Geometry check sheet. Reference: the model listing, model coordinates, mm. A direction names the side the tool comes from. Round coordinates to 2 decimals unless told otherwise and drop trailing zeros. Order: outer loops, then holes, each group sorted by start corner. A loop starts at its lowest first (then second) coordinate and runs counter-clockwise, first axis right, second up.
(1) Sectioned sample at B-B (x = -21.5). Record the boundary of the cut face in (y, z) (1 decimal).
(2) Material ranges on line 1 along X through (y, z) = (12.25, -2); line 2 along Z through (x, y) = (-12.5, 1.75); line 3 along Y through (x, z) = (-1, -0.5) (1 decimal), recorded low to high.
(3) Sectioned sample at A-A (x = 11). Record the boundary of the cut face in (y, z) (1 decimal).
(4) Release check for a two-part mould opening along Z. For faces 1 (the face through (-22.86, 2, -5)), 2 (the face through (0, 25.4, -9)), 3 (the face through (0, 13, 12.7)), 4 (the face through (-22.06, 24.62, -9.27)) record: +Z half, -Z half, draft (parallel to the pull), parting line (faces both ways), or undercut.
(5) Set-up check for faces 5 (the face through (-21.867, 1.61, -9.218)), 6 (the face through (-20.326, 24.617, 8.73)), 7 (the face through (-0.2, 13.95, -4.56)): record each of +Z, -Z, +X, -X, +Y, -Y from which the full face is reachable in a straight line by a thin tool's end or side.
(6) Go/stop test with flat-tipped pins: pin 1 (10 mm diameter, centred on x = -7.5, z = -2, fed in from -Y) (3 decimals); pin 2 (1.5 mm diameter, centred on x = 6.65, z = -0.77, fed in from +Y); pin 3 (0.9 mm diameter, centred on x = -24.5, y = 2, fed in from +Z). Record where each tip stops, or that it passes through.
from build123d import *

# Parameters (mm, degrees)
SKETCH1_W           = 50.8
SKETCH1_H           = 25.4
BOSS_EXTRUDE1_DEPTH = 25.4
SKETCH6_R           = 0.635
CUT_EXTRUDE1_DEPTH  = 39.1
CUT_EXTRUDE2_DEPTH  = 1.5875
CUT_EXTRUDE3_DEPTH  = 3.175
FILLET1_R           = 3.302
FILLET2_R           = 0.8128
CHAMFER1_SIZE       = 0.635
FILLET3_R           = 1.5875


with BuildPart() as part:
    # Sketch1 → Boss-Extrude1 (new body)
    with BuildSketch(Plane(origin=(0, 0, 0), x_dir=(1, 0, 0), z_dir=(0, 1, 0))):
        Rectangle(SKETCH1_W, SKETCH1_H)
    extrude(amount=BOSS_EXTRUDE1_DEPTH)

    # Sketch6 → Cut-Extrude1 (cut, through all)
    with BuildSketch(Plane(origin=(0, 25.4, 0), x_dir=(1, 0, 0), z_dir=(0, 1, 0))):
        with Locations(Location((-5.6134, 1.4605, 0), (0, 0, 270))):
            Circle(SKETCH6_R)
        with Locations(Location((-0.2286, 3.9243, 0), (0, 0, 270))):
            Circle(SKETCH6_R)
        with Locations(Location((-0.2032, 2.3241, 0), (0, 0, 270))):
            Circle(SKETCH6_R)
        with Locations(Location((-4.1402, -5.0927, 0), (0, 0, 270))):
            Circle(SKETCH6_R)
        with Locations(Location((-8.7376, -5.3467, 0), (0, 0, 270))):
            Circle(SKETCH6_R)
        with Locations(Location((6.6548, 0.7747, 0), (0, 0, 270))):
            Circle(SKETCH6_R)
        with Locations(Location((8.2804, 3.1369, 0), (0, 0, 270))):
            Circle(SKETCH6_R)
        with Locations(Location((-3.3782, 0.0635, 0), (0, 0, 270))):
            Circle(SKETCH6_R)
    extrude(amount=-CUT_EXTRUDE1_DEPTH, mode=Mode.SUBTRACT)

    # Sketch7 → Cut-Extrude2 (cut)
    with BuildSketch(Plane(origin=(0, 25.4, 0), x_dir=(1, 0, 0), z_dir=(0, 1, 0))):
        with BuildLine():
            Line((-20.955, -7.024066704), (-20.955, 7.024066704))
            Line((-20.955, 7.024066704), (-22.046716648, 8.115783352))
            ThreePointArc((-22.046716648, 8.115783352), (-22.046716648, 9.283216648), (-20.879283352, 9.283216648))
            Line((-20.879283352, 9.283216648), (-19.787566704, 8.1915))
            Line((-19.787566704, 8.1915), (20.168566704, 8.1915))
            Line((20.168566704, 8.1915), (21.260283352, 9.283216648))
            ThreePointArc((21.260283352, 9.283216648), (22.427716648, 9.283216648), (22.427716648, 8.115783352))
            Line((22.427716648, 8.115783352), (21.336, 7.024066704))
            Line((21.336, 7.024066704), (21.336, -7.024066704))
            Line((21.336, -7.024066704), (22.427716648, -8.115783352))
            ThreePointArc((22.427716648, -8.115783352), (22.427716648, -9.283216648), (21.260283352, -9.283216648))
            Line((21.260283352, -9.283216648), (20.168566704, -8.1915))
            Line((20.168566704, -8.1915), (-19.787566704, -8.1915))
            Line((-19.787566704, -8.1915), (-20.879283352, -9.283216648))
            ThreePointArc((-20.879283352, -9.283216648), (-22.046716648, -9.283216648), (-22.046716648, -8.115783352))
            Line((-22.046716648, -8.115783352), (-20.955, -7.024066704))
        make_face()
    extrude(amount=-CUT_EXTRUDE2_DEPTH, mode=Mode.SUBTRACT)

    # Sketch8 → Cut-Extrude3 (cut)
    with BuildSketch(Plane.XZ):
        Polygon((22.86, 10.16), (-22.86, 10.16), (-22.86, 3.175), (-25.4, 3.175), (-25.4, -3.175), (-22.86, -3.175), (-22.86, -10.16), (22.86, -10.16), align=None)
    extrude(amount=-CUT_EXTRUDE3_DEPTH, mode=Mode.SUBTRACT)

    # Fillet1
    fillet1_edges = [part.edges().sort_by_distance(p)[0] for p in [
        (22.86, 1.5875, 10.16),
        (22.86, 1.5875, -10.16),
        (-22.86, 1.5875, -10.16),
        (-22.86, 1.5875, 10.16),
    ]]
    fillet(fillet1_edges, radius=FILLET1_R)

    # Fillet2
    fillet2_edges = [part.edges().sort_by_distance(p)[0] for p in [
        (-22.86, 1.5875, -3.175),
        (-22.86, 1.5875, 3.175),
    ]]
    fillet(fillet2_edges, radius=FILLET2_R)

    # Chamfer1
    # the kernel refuses this chamfer: 0.635 mm, written as the material it takes off along each edge
    with BuildSketch(Plane(origin=(-5.6134, 3.175, -1.4605), x_dir=(0, 0, 1), z_dir=(-1, 0, 0))) as chamfer1_piece_1:
        Polygon((0.635 + CHAMFER1_SIZE, 0), (0.635, CHAMFER1_SIZE), (0.635, 0), align=None)
    revolve(axis=Axis((-5.6134, 3.175, -1.4605), (0, 1, 0)), mode=Mode.SUBTRACT)
    with BuildSketch(Plane(origin=(-0.2286, 3.175, -3.9243), x_dir=(0, 0, 1), z_dir=(-1, 0, 0))) as chamfer1_piece_2:
        Polygon((0.635 + CHAMFER1_SIZE, 0), (0.635, CHAMFER1_SIZE), (0.635, 0), align=None)
    revolve(axis=Axis((-0.2286, 3.175, -3.9243), (0, 1, 0)), mode=Mode.SUBTRACT)
    with BuildSketch(Plane(origin=(-0.2032, 3.175, -2.3241), x_dir=(0, 0, 1), z_dir=(-1, 0, 0))) as chamfer1_piece_3:
        Polygon((0.635 + CHAMFER1_SIZE, 0), (0.635, CHAMFER1_SIZE), (0.635, 0), align=None)
    revolve(axis=Axis((-0.2032, 3.175, -2.3241), (0, 1, 0)), mode=Mode.SUBTRACT)
    with BuildSketch(Plane(origin=(-4.1402, 3.175, 5.0927), x_dir=(0, 0, 1), z_dir=(-1, 0, 0))) as chamfer1_piece_4:
        Polygon((0.635 + CHAMFER1_SIZE, 0), (0.635, CHAMFER1_SIZE), (0.635, 0), align=None)
    revolve(axis=Axis((-4.1402, 3.175, 5.0927), (0, 1, 0)), mode=Mode.SUBTRACT)
    with BuildSketch(Plane(origin=(-8.7376, 3.175, 5.3467), x_dir=(0, 0, 1), z_dir=(-1, 0, 0))) as chamfer1_piece_5:
        Polygon((0.635 + CHAMFER1_SIZE, 0), (0.635, CHAMFER1_SIZE), (0.635, 0), align=None)
    revolve(axis=Axis((-8.7376, 3.175, 5.3467), (0, 1, 0)), mode=Mode.SUBTRACT)
    with BuildSketch(Plane(origin=(6.6548, 3.175, -0.7747), x_dir=(0, 0, 1), z_dir=(-1, 0, 0))) as chamfer1_piece_6:
        Polygon((0.635 + CHAMFER1_SIZE, 0), (0.635, CHAMFER1_SIZE), (0.635, 0), align=None)
    revolve(axis=Axis((6.6548, 3.175, -0.7747), (0, 1, 0)), mode=Mode.SUBTRACT)
    with BuildSketch(Plane(origin=(8.2804, 3.175, -3.1369), x_dir=(0, 0, 1), z_dir=(-1, 0, 0))) as chamfer1_piece_7:
        Polygon((0.635 + CHAMFER1_SIZE, 0), (0.635, CHAMFER1_SIZE), (0.635, 0), align=None)
    revolve(axis=Axis((8.2804, 3.175, -3.1369), (0, 1, 0)), mode=Mode.SUBTRACT)
    with BuildSketch(Plane(origin=(-3.3782, 3.175, -0.0635), x_dir=(0, 0, 1), z_dir=(-1, 0, 0))) as chamfer1_piece_8:
        Polygon((0.635 + CHAMFER1_SIZE, 0), (0.635, CHAMFER1_SIZE), (0.635, 0), align=None)
    revolve(axis=Axis((-3.3782, 3.175, -0.0635), (0, 1, 0)), mode=Mode.SUBTRACT)

    # Fillet3
    fillet3_edges = [part.edges().sort_by_distance(p)[0] for p in [
        (-25.4, 12.7, -12.7),
        (25.4, 12.7, -12.7),
        (25.4, 12.7, 12.7),
        (-25.4, 12.7, 12.7),
    ]]
    fillet(fillet3_edges, radius=FILLET3_R)


solid = part.part
Answer below:
1. outline: (0, -12.7) - (25.4, -12.7) - (25.4, -9.5) - (23.8, -9.5) - (23.8, -7.6) - (25.4, -7.6) - (25.4, 7.6) - (23.8, 7.6) - (23.8, 9.5) - (25.4, 9.5) - (25.4, 12.7) - (0, 12.7) - (0, 9.5) - (3.2, 9.5) - (3.2, -9.5) - (0, -9.5) - close
2. line 1: x = -25.4 to -5.95, -5.28 to -0.75, 0.34 to 25.4
2. line 2: z = -12.7 to -10.16, 10.16 to 12.7
2. line 3: y = 3.2 to 23.8
3. outline: (0, -12.7) - (25.4, -12.7) - (25.4, -8.2) - (23.8, -8.2) - (23.8, 8.2) - (25.4, 8.2) - (25.4, 12.7) - (0, 12.7) - (0, 10.2) - (3.2, 10.2) - (3.2, -10.2) - (0, -10.2) - close
4. face 1: undercut
4. face 2: draft
4. face 3: +Z half
4. face 4: undercut
5. face 5: -Y
5. face 6: +Y
5. face 7: +Y, -Y
6. pin 1: stops at y = 3.175
6. pin 2: stops at y = 23.81
6. pin 3: stops at z = 12.68
